Autodesk Fusion 360 part; units mm, degrees
sketch "Sketch1" plane through (0, 0, 0) normal (0, 0, 1) x (1, 0, 0)
  line L0 (-25.748, 28.7303) -> (11.9841, 36.6874)
  line L1 (11.9841, 36.6874) -> (37.7548, 7.9326)
  line L2 (37.7548, 7.9326) -> (25.748, -28.7303)
  line L3 (25.748, -28.7303) -> (-11.9841, -36.6874)
  line L4 (-11.9841, -36.6874) -> (-37.7548, -7.9326)
  line L5 (-37.7548, -7.9326) -> (-25.748, 28.7303)
  line L6 (-25.748, 28.7303) -> (25.748, -28.7303) construction
  dimension "d1" = 38.562
  dimension "d2" = 38.562
  dimension "d3" = 38.613
  dimension "d4" = 38.613
  dimension "d5" = 38.579
  dimension "d6" = 38.579
  dimension "d7" = 66.85
  dimension "d8" = 66.82
extrude "Extrude1" add sketch "Sketch1" along normal blind 2.5
sketch "Sketch2" plane through (0, 0, 2.5) normal (0, 0, 1) x (-1, 0, 0)
  line L0 (37.7548, 7.9326) -> (11.9841, 36.6874)
  line L1 (11.9841, 36.6874) -> (-25.748, 28.7303)
  line L2 (-25.748, 28.7303) -> (-37.7548, -7.9326)
  line L3 (-37.7548, -7.9326) -> (-11.9841, -36.6874)
  line L4 (-11.9841, -36.6874) -> (25.748, -28.7303)
  line L5 (25.748, -28.7303) -> (37.7548, 7.9326)
  circle A0 centre (0, 0) radius 16.5
  dimension "d11" = 33
extrude "Extrude2" add sketch "Sketch2" along normal blind 4 draft -45 contours A0
sketch "Sketch3" plane through (0, 0, 6.5) normal (0, 0, 1) x (-1, 0, 0)
  circle A0 centre (0, 0) radius 12.5
  circle A1 centre (0, 0) radius 10
  circle A2 centre (0, 0) radius 12.5
  dimension "d14" = 20
  dimension "d15" = 25
extrude "Extrude3" add sketch "Sketch3" along normal blind 8.5
Can you work these out from the model? Positions are in its coordinate system, mm. A direction names the side the tool comes from. Give positions to 0.01 mm unless a question says otherwise; leave off trailing zeros. Loops run counter-clockwise (first coordinate to the right, second up) from the corner with the lowest first, then second, coordinate; pieces in that order, holes last. Notation, with made-up numbers: (-22, -31.75) - (-9, -31.75) arc R21 ccw to (-9, -13.75) - close; hole circle Ø5 at (-39.5, -38). An arc over 180 degrees is marked (long way). One line per item, written item: value.
(1) If we section it at A-A, the plane z = 4.5: List the corners of the cut face in (x, y) for me, plus the area to 3 significant figures.
Verdict:
outline: circle Ø29 at (0, 0)
area: 661 mm^2
(2) On a 3-axis mill with a long thin cutter (end or side, diameter ignored), from which of +Z, -Z, +X, -X, +Y, -Y can I reach the whole of each face in a straight line? I mean faces 1 (the face through (-24.7, -22.5, 1.2)), 2 (the face through (-11.923, 3.755, 10.69)). Say none if no direction works.
Verdict:
face 1: +Z, -Z, -X, -Y
face 2: +Z
(3) I need wall thicknesses on line 1 along X through (y, z) = (0, 8.5); line 2 along Z through (x, y) = (-4, -6). Which ranges of each line are inside material? Lowest first, please.
Verdict:
line 1: -12.5 to -10, 10 to 12.5
line 2: 0 to 6.5
(4) If we section it at D-D, the plane y = 30.5: List the corners of the cut face in (x, z) for me.
Verdict:
outline: (-17.36, 0) - (17.53, 0) - (17.53, 2.5) - (-17.36, 2.5) - close
(5) If we section it at C-C, the plane y = 0: List the corners of the cut face in (x, z) for me, plus the area to 3 significant figures.
Verdict:
outline: (-35.16, 0) - (35.16, 0) - (35.16, 2.5) - (16.5, 2.5) - (12.5, 6.5) - (12.5, 15) - (10, 15) - (10, 6.5) - (-10, 6.5) - (-10, 15) - (-12.5, 15) - (-12.5, 6.5) - (-16.5, 2.5) - (-35.16, 2.5) - close
area: 334 mm^2
(6) If we section it at B-B, the plane x = 0: List the corners of the cut face in (y, z) for me, plus the area to 3 significant figures.
Verdict:
outline: (-34.16, 0) - (34.16, 0) - (34.16, 2.5) - (16.5, 2.5) - (12.5, 6.5) - (12.5, 15) - (10, 15) - (10, 6.5) - (-10, 6.5) - (-10, 15) - (-12.5, 15) - (-12.5, 6.5) - (-16.5, 2.5) - (-34.16, 2.5) - close
area: 329 mm^2
(7) If we mould it in two halves opening along Y, with no side actions, what happens to faces 3 (the face through (7.146, -32.653, 1.232)), 4 (the face through (-7.146, 32.653, 1.232)), 5 (the face through (0, 0, 6.5))? For each: released by +Y, released by -Y, zero draft, split by the parting line, or undercut.
Verdict:
face 3: released by -Y
face 4: released by +Y
face 5: undercut
(8) I'm going to push flat-ended pins straight in: pin 1 (16 mm diameter, centred on x = -2.5, y = 3.5, fed in from +Z); pin 2 (1.5 mm diameter, centred on x = -14, z = 9, fed in from -Y); pin 3 (8 mm diameter, centred on y = -17, z = 3.5, fed in from +X); pin 4 (8 mm diameter, centred on y = -2, z = 1.5, fed in from -X). Where does each tip first touch, or does it pass through?
Verdict:
pin 1: z = 15
pin 2: through
pin 3: x = 30.86
pin 4: x = -37.12
